from build123d import *

# Parameters (mm, degrees)
F1_DEPTH  = 16.1798
F2_W      = 14.6956490017
F2_H      = 39.0100460752
F3_DEPTH  = 25.4
F4_W      = 7.289106492
F4_H      = 24.3518359493
F5_DEPTH  = 6.0198
F6_W      = 0.4318
F6_H      = 1.4841509983
F7_DEPTH  = 2.54
F8_W      = 1.707770396
F8_H      = 26.8365105148
F9_DEPTH  = 5.8674
F10_W     = 4.3080397882
F10_H     = 25.773898873
F11_DEPTH = 8.382
F12_W     = 0.4299804568
F12_H     = 1.4841509983
F13_DEPTH = 1.4986
F14_W     = 0.3396534594
F14_H     = 2.54
F14_W_2   = 0.0413465406
F15_DEPTH = 25.4
F16_R     = 0.5


with BuildPart() as f1:
    # F0 (on Front) → F1 (new body)
    with BuildSketch(Plane.XZ):
        Polygon((7.4940245816, -8.5250653475), (7.4940245816, 30.4849807278), (-1.3047935208, 25.4049807278), (-1.3047935208, -3.4450653475), align=None)
    extrude(amount=F1_DEPTH)

    # F2 (on face) → F3 (cut)
    with BuildSketch(Plane.YZ.offset(7.4940245816)):
        with Locations((-8.8319754991, 10.9799576901)):
            Rectangle(F2_W, F2_H)
    extrude(amount=-F3_DEPTH, mode=Mode.SUBTRACT)

    # F4 (on face) → F5 (cut)
    with BuildSketch(Plane.XZ):
        with Locations((4.2547506746, 11.1802831525)):
            Rectangle(F4_W, F4_H)
    extrude(amount=F5_DEPTH, mode=Mode.SUBTRACT)

    # F6 (on face) → F7 (cut)
    with BuildSketch(Plane(origin=(-1.8179554345, 0, -3.1487911785), x_dir=(0.8660254038, 0, -0.5), z_dir=(-0.5, 0, -0.8660254038))):
        with Locations((7.5819472408, 0.7420754991)):
            Rectangle(F6_W, F6_H)
    extrude(amount=-F7_DEPTH, mode=Mode.SUBTRACT)

    # F8 (on Front) → F9 (cut)
    with BuildSketch(Plane.XZ):
        with Locations((7.0332919713, 12.55759981)):
            Rectangle(F8_W, F8_H)
    extrude(amount=F9_DEPTH, mode=Mode.SUBTRACT)

    # F10 (on Front) → F11 (cut)
    with BuildSketch(Plane.XZ):
        with Locations((8.7046686094, 13.3732402755)):
            Rectangle(F10_W, F10_H)
    extrude(amount=F11_DEPTH, mode=Mode.SUBTRACT)

    # F12 (on face) → F13 (cut)
    with BuildSketch(Plane(origin=(-11.3268777267, 0, 19.6187277137), x_dir=(0.8660254038, 0, 0.5), z_dir=(-0.5, 0, 0.8660254038))):
        with Locations((18.6048597097, -0.7420754991)):
            Rectangle(F12_W, F12_H)
    extrude(amount=-F13_DEPTH, mode=Mode.SUBTRACT)

    # F14 (on face) → F15 (cut)
    with BuildSketch(Plane.YZ.offset(0.6101974286)):
        with Locations((-1.3143242686, 19.5710362089)):
            Rectangle(F14_W, F14_H)
        with Locations((-1.5048242686, 19.5710362089)):
            Rectangle(F14_W_2, F14_H)
    extrude(amount=-F15_DEPTH, mode=Mode.SUBTRACT)

    # F16
    f16_edges = [f1.edges().sort_by_distance(p)[0] for p in [
        (7.494025, -0.742075, 30.484981),
        (7.494025, -0.742075, -8.525065),
        (-1.304794, -0.742075, -3.445065),
        (-1.304794, -0.742075, 25.404981),
        (7.494025, -0.742075, 26.26019),
    ]]
    fillet(f16_edges, radius=F16_R)


solid = f1.part
Build history of the part. All positions in model axes, mm. A direction names the side the tool comes from. Round coordinates to 2 decimals unless told otherwise and drop trailing zeros. Write each loop counter-clockwise with the first axis right and the second up, starting at its lowest first coordinate (ties: lowest second). Pieces come first, ordered by that corner, then holes. Notation, with made-up numbers: M 68,30 L 96,30 A21 cw 96,41 Z; hole C -8,-38 d9. An arc over 180 degrees is marked long. Answer as a JSON object with one key per item and string values. Group by question number.
(1) Which spindle directions (+Z, -Z, +X, -X, +Y, -Y) get a long thin tool onto all of the face, cutting with end or side? Do faces 5 (the flat face through (4.97, -0.75, 28.17)), 6 (the flat face through (4, -1, -0.996)), 7 (the flat face through (0, 0, 11)). Say none if no direction does.
(2) Flat gauge pins, fed straight in: pin 1 (1 mm diameter, centred on x = -0.5, z = 19, fed in from -Y); pin 2 (3 mm diameter, centred on x = 2.5, z = 9, fed in from +Y); pin 3 (0.7 mm diameter, centred on y = -1, z = 24.5, fed in from +X). Where does each tip first touch, or does it go through?
(3) Mould opens along Z. For faces 1 (the flat face through (3, -1.484, 25)), 2 (the flat face through (5.827, -0.732, -7.563)), 3 (the flat face through (0.61, -1, 11)), 4 (the flat face through (5.561, -0.732, -5.963)) say: pulls with the +Z half, pulls with the -Z half, needs draft (parallel to the pull), parting line crosses it, or undercut.
(4) Cut at A-A (y = -0.4). Give the cut face in (x, z), and give its area (3 significant figures).
(5) Cut at C-C (z = -6). Give the cut face in (x, y).
(6) Cut at D-D (z = 23). Give the cut face in (x, y).
(7) Drill centre lines: L1, parallel to Z at x = 7, y = -0.8; L2, parallel to Z at x = 6.75, y = -1.3; L3, parallel to Z at x = 6, y = -1.05. Where is each one in solid material? Low to high.
(8) Cut at B-B (x = 3). Give the cut face in (y, z), and give its area (3 significant figures).
Responses:
{
 "1": {"face 5": "+Y, -Y", "face 6": "+X, +Y, -Y", "face 7": "+Z, -Z, +X, -X, +Y"},
 "2": {"pin 1": "stops at y = -1.14", "pin 2": "passes through", "pin 3": "stops at x = 6.18"},
 "3": {"face 1": "needs draft", "face 2": "pulls with the -Z half", "face 3": "undercut", "face 4": "undercut"},
 "4": {"outline": "M -1.3,-3.16 A0.5 ccw -1.05,-3.59 L 4.56,-6.83 L 5.83,-4.63 L 6.21,-4.85 L 4.94,-7.05 L 6.74,-8.09 A0.5 ccw 7.49,-7.66 L 7.49,-1 L 0.61,-1 L 0.61,23.36 L 6.18,23.36 L 6.18,25.98 L 6.55,25.98 L 6.55,26.26 L 6.99,26.26 A0.5 ccw 7.49,26.76 L 7.49,29.62 A0.5 ccw 6.74,30.05 L 4.97,29.03 L 5.72,27.73 L 5.35,27.52 L 4.6,28.81 L -1.05,25.55 A0.5 ccw -1.3,25.12 Z", "area": "125 mm2"},
 "5": {"outline": "M 3.12,-1.48 L 5.04,-1.48 L 5.04,0 L 3.12,0 Z; M 5.54,-1.48 L 7.49,-1.48 L 7.49,0 L 5.54,0 Z"},
 "6": {"outline": "M -1.3,-1.48 L 0.61,-1.48 L 0.61,0 L -1.3,0 Z"},
 "7": {"L1": "z = -8.16 to -1, 26.26 to 30.12", "L2": "z = -8.1 to -1, 26.26 to 30.06", "L3": "z = -7.66 to -5.2, -4.73 to -1, 23.36 to 29.62"},
 "8": {"outline": "M -1.48,-5.93 L 0,-5.93 L 0,-1 L -1.48,-1 Z; M -1.48,23.36 L 0,23.36 L 0,27.89 L -1.48,27.89 Z", "area": "14.1 mm2"}
}
